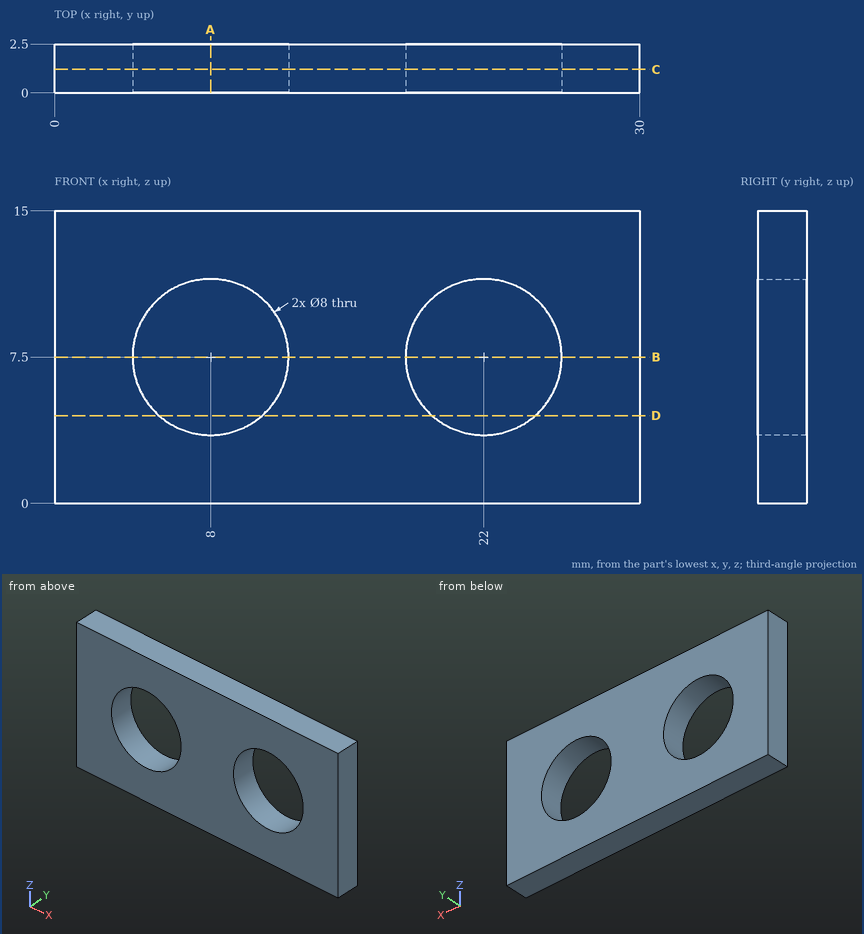
Source: three-view drawing plus pictorial views. Frame: mm from the lowest corner of the part. Give positions to 0.01 mm unless a question says otherwise; leave off trailing zeros. Write each loop counter-clockwise with the first axis right and the second up, starting at its lowest first coordinate (ties: lowest second). Pieces come first, ordered by that corner, then holes. Notation, with made-up numbers: (68, -21) -> (105, -21) arc R26 cw to (105, 10) -> close; hole circle Ø1 at (-33.75, 27). An arc over 180 degrees is marked (long way). Answer in a Markdown table with one row per item.
(1) Section query B-B on z = 7.5. Return loops of the section in (x, y).
Answers below:
| item | result |
|---|---|
| outline | (0, 0) -> (4, 0) -> (4, 2.5) -> (0, 2.5) -> close; (12, 0) -> (18, 0) -> (18, 2.5) -> (12, 2.5) -> close; (26, 0) -> (30, 0) -> (30, 2.5) -> (26, 2.5) -> close |
(2) Section query A-A on x = 8. Return loops of the section in (y, z).
Answers below:
| item | result |
|---|---|
| outline | (0, 0) -> (2.5, 0) -> (2.5, 3.5) -> (0, 3.5) -> close; (0, 11.5) -> (2.5, 11.5) -> (2.5, 15) -> (0, 15) -> close |
(3) Pin query (flat end, axial travel): pin 1 (1 mm diameter, centred on x = 6.5, z = 9, fed in from +Y). Return the tip coordinate at first contact, or that it passes through.
Answers below:
| item | result |
|---|---|
| pin 1 | through |
(4) Section query D-D on z = 4.5. Return loops of the section in (x, y).
Answers below:
| item | result |
|---|---|
| outline | (0, 0) -> (5.35, 0) -> (5.35, 2.5) -> (0, 2.5) -> close; (10.65, 0) -> (19.35, 0) -> (19.35, 2.5) -> (10.65, 2.5) -> close; (24.65, 0) -> (30, 0) -> (30, 2.5) -> (24.65, 2.5) -> close |
(5) Ray query, line 1 along X through (y, z) = (1, 7.5); line 2 along Z through (x, y) = (22, 1); line 3 along X through (y, z) = (0.4, 8.75). Return the intervals inside material, ascending. Write a range as [from, to].
Answers below:
| item | result |
|---|---|
| line 1 | [0, 4], [12, 18], [26, 30] |
| line 2 | [0, 3.5], [11.5, 15] |
| line 3 | [0, 4.2], [11.8, 18.2], [25.8, 30] |
(6) Section query C-C on y = 1.2. Return loops of the section in (x, z).
Answers below:
| item | result |
|---|---|
| outline | (0, 0) -> (30, 0) -> (30, 15) -> (0, 15) -> close; hole circle Ø8 at (8, 7.5); hole circle Ø8 at (22, 7.5) |
